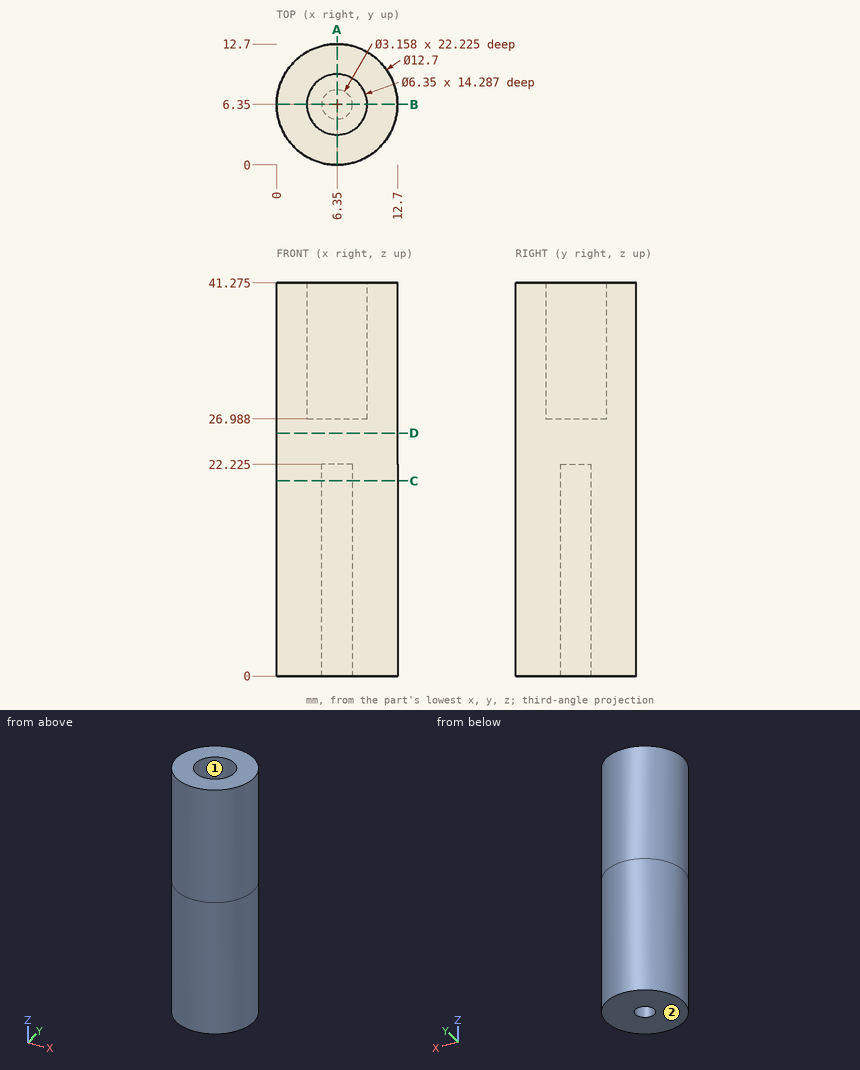
Part print with two shaded views. Sizes in mm from the minimum x, y, z corner. Round coordinates to 2 decimals unless told otherwise and drop trailing zeros. Loops run counter-clockwise (first coordinate to the right, second up) from the corner with the lowest first, then second, coordinate; pieces in that order, holes last.
1. Slice it at A-A (x = 6.35). Give the cut face in (y, z) (1 decimal).
Solutions:
outline: (0, 0) - (4.8, 0) - (4.8, 22.2) - (7.9, 22.2) - (7.9, 0) - (12.7, 0) - (12.7, 41.3) - (9.5, 41.3) - (9.5, 27) - (3.2, 27) - (3.2, 41.3) - (0, 41.3) - close
2. Slice it at D-D (z = 25.5). Give the cut face in (x, y).
Solutions:
outline: circle Ø12.7 at (6.35, 6.35)
3. Drill centre lines: line 1 along Y through (x, z) = (6.35, 6); line 2 along Z through (x, y) = (7.75, 9); line 3 along Y through (x, z) = (6.35, 37.5) (1 decimal). Where is each one in solid material? Low to high.
Solutions:
line 1: y = 0 to 4.77, 7.93 to 12.7
line 2: z = 0 to 26.99
line 3: y = 0 to 3.2, 9.5 to 12.7
4. Two-plate mould, pull along Y, no slides. Class the marked faces 1 and 2: pulls with the +Y half, pulls with the -Y half, needs draft (parallel to the pull), parting line crosses it, or undercut.
Solutions:
face 1: undercut
face 2: needs draft
5. Flat gauge pins, fed straight in: pin 1 (1.5 mm diameter, centred on x = 11.5, z = 18.5, fed in from +Y); pin 2 (3 mm diameter, centred on x = 6.5, y = 5, fed in from +Z); pin 3 (4 mm diameter, centred on y = 10.5, z = 25.5, fed in from -X) (1 decimal). Where does each tip first touch, or does it go through?
Solutions:
pin 1: stops at y = 10.93
pin 2: stops at z = 26.99
pin 3: stops at x = 0.4
6. Slice it at C-C (z = 20.5). Give the cut face in (x, y).
Solutions:
outline: circle Ø12.7 at (6.35, 6.35); hole circle Ø3.16 at (6.35, 6.35)
